```python
from build123d import *

# Parameters (mm, degrees)
SKETCH_1_R          = 8
SKETCH_1_R_2        = 4
EXTRUDE_1_DEPTH     = 3.8
SKETCH_4_W          = 6
SKETCH_4_H          = 6
EXTRUDE_2_DEPTH     = 3.8
SKETCH_5_R          = 2
CUT_EXTRUDE_3_DEPTH = 1
SKETCH_6_R          = 1
CUT_EXTRUDE_4_DEPTH = 15.691494138
CUT_EXTRUDE_5_DEPTH = 15.91442255


with BuildPart() as part:
    # 草图1 → 凸台-拉伸1 (new body)
    with BuildSketch(Plane(origin=(0, 0, 0), x_dir=(1, 0, 0), z_dir=(0, 1, 0))):
        with Locations(Location((0, 0, 0), (0, 0, 90))):
            Circle(SKETCH_1_R)
        with Locations(Location((0, 0, 0), (0, 0, 90))):
            Circle(SKETCH_1_R_2, mode=Mode.SUBTRACT)
    extrude(amount=EXTRUDE_1_DEPTH)

    # 草图4 → 凸台-拉伸2 (add)
    with BuildSketch(Plane(origin=(0, 3.8, 0), x_dir=(1, 0, 0), z_dir=(0, 1, 0))):
        with Locations((-9, 0)):
            Rectangle(SKETCH_4_W, SKETCH_4_H)
        with Locations((9, 0)):
            Rectangle(SKETCH_4_W, SKETCH_4_H)
    extrude(amount=-EXTRUDE_2_DEPTH)

    # 草图5 → 切除-拉伸3 (cut)
    with BuildSketch(Plane.XZ):
        with Locations(Location((-9.5, 0, 0), (0, 0, 270))):
            Circle(SKETCH_5_R)
        with Locations(Location((9.5, 0, 0), (0, 0, 90))):
            Circle(SKETCH_5_R)
    extrude(amount=-CUT_EXTRUDE_3_DEPTH, mode=Mode.SUBTRACT)

    # 草图6 → 切除-拉伸4 (cut, through all)
    with BuildSketch(Plane.XZ.offset(-1)):
        with Locations(Location((-9.5, 0, 0), (0, 0, 270))):
            Circle(SKETCH_6_R)
        with Locations(Location((9.5, 0, 0), (0, 0, 90))):
            Circle(SKETCH_6_R)
    extrude(amount=-CUT_EXTRUDE_4_DEPTH, mode=Mode.SUBTRACT)

    # 草图7 → 切除-拉伸5 (cut, through all)
    with BuildSketch(Plane(origin=(0, 3.8, 0), x_dir=(1, 0, 0), z_dir=(0, 1, 0))):
        with BuildLine():
            Line((-4.05, 6.899094143), (-2.8, 4.734030634))
            Line((-2.8, 4.734030634), (-2.8, 2.856571371))
            ThreePointArc((-2.8, 2.856571371), (0, 4), (2.8, 2.856571371))
            Line((2.8, 2.856571371), (2.8, 4.734030634))
            Line((2.8, 4.734030634), (4.05, 6.899094143))
            ThreePointArc((4.05, 6.899094143), (0, 8), (-4.05, 6.899094143))
        make_face()
    extrude(amount=-CUT_EXTRUDE_5_DEPTH, mode=Mode.SUBTRACT)


solid = part.part
```
Check sheet for the modelled part. Datum: model origin and axes. Units: mm. A direction names the side the tool comes from. Round coordinates to 2 decimals unless told otherwise and drop trailing zeros. Loops run counter-clockwise (first coordinate to the right, second up) from the corner with the lowest first, then second, coordinate; pieces in that order, holes last. Notation, with made-up numbers: (45, 62.25) -> (53, 62.25) arc R15 ccw to (53, 88.25) -> close; hole circle Ø9 at (66.25, -13). An arc over 180 degrees is marked (long way). Write item = value, one per line. Start each with the question number.
1) Sectioned sample at A-A, the plane z = 0. Record the cut outline in (x, y), plus the area to 3 significant figures.
2) Set-up check for faces 1 (the flat face through (-10, 2, -3)), 2 (the flat face through (10, 2, 3)), 3 (the flat face through (-10, 2, 3)): record each of +Z, -Z, +X, -X, +Y, -Y from which the full face is reachable in a straight line by a thin tool's end or side.
3) Sectioned sample at B-B, the plane x = -9.5. Record the cut outline in (y, z).
4) Gauge pin test, flat ends, axial feed: pin 1 Ø1.1 at (x, y) = (10.5, 2) entering from +Z; pin 2 Ø5 at (x, z) = (9.5, 0) entering from +Y; pin 3 Ø2 at (y, z) = (1.5, -4.5) entering from -X; pin 4 Ø1.2 at (x, z) = (9, 0.5) entering from -Y. Record the tip position at first contact, or that the pin passes through.
5) Thickness scan on probe 1 along X at (y, z) = (0.5, 0); probe 2 along X at (y, z) = (2.2, 0); probe 3 along Z at (x, y) = (9.25, 1.55). Record the ranges inside material, lowest first.
6) Sectioned sample at C-C, the plane y = 1.7. Record the cut outline in (x, z).
7) Release check for a two-part mould opening along Z. For faces 4 (the cylindrical face through (0, 2, 4)), 5 (the flat face through (-2.8, 2, -4)), 6 (the flat face through (-10.4, 1, -0.9)), 7 (the flat face through (-3.434, 1.927, -5.832)) record: released by +Z, released by -Z, zero draft, split by the parting line, or undercut.
8) Sectioned sample at D-D, the plane z = -3.75. Record the cut outline in (x, y).
Results are:
q1.outline = (-12, 0) -> (-11.5, 0) -> (-11.5, 1) -> (-10.5, 1) -> (-10.5, 3.8) -> (-12, 3.8) -> close; (-8.5, 1) -> (-7.5, 1) -> (-7.5, 0) -> (-4, 0) -> (-4, 3.8) -> (-8.5, 3.8) -> close; (4, 0) -> (7.5, 0) -> (7.5, 1) -> (8.5, 1) -> (8.5, 3.8) -> (4, 3.8) -> close; (10.5, 1) -> (11.5, 1) -> (11.5, 0) -> (12, 0) -> (12, 3.8) -> (10.5, 3.8) -> close
q1.area = 41.6 mm^2
q2.face_1 = -Z, -X, +Y, -Y
q2.face_2 = +Z, +X, +Y, -Y
q2.face_3 = +Z, -X, +Y, -Y
q3.outline = (0, -3) -> (3.8, -3) -> (3.8, -1) -> (1, -1) -> (1, -2) -> (0, -2) -> close; (0, 2) -> (1, 2) -> (1, 1) -> (3.8, 1) -> (3.8, 3) -> (0, 3) -> close
q4.pin_1 = 3
q4.pin_2 = 3.8
q4.pin_3 = -7.19
q4.pin_4 = 1
q5.probe_1 = -12 to -11.5, -7.5 to -4, 4 to 7.5, 11.5 to 12
q5.probe_2 = -12 to -10.5, -8.5 to -4, 4 to 8.5, 10.5 to 12
q5.probe_3 = -3 to -0.97, 0.97 to 3
q6.outline = (-12, -3) -> (-7.42, -3) arc R8 ccw to (-4.05, -6.9) -> (-2.8, -4.73) -> (-2.8, -2.86) arc R4 cw (long way) to (2.8, -2.86) -> (2.8, -4.73) -> (4.05, -6.9) arc R8 ccw to (7.42, -3) -> (12, -3) -> (12, 3) -> (7.42, 3) arc R8 ccw to (-7.42, 3) -> (-12, 3) -> close; hole circle Ø2 at (-9.5, 0); hole circle Ø2 at (9.5, 0)
q7.face_4 = undercut
q7.face_5 = zero draft
q7.face_6 = undercut
q7.face_7 = released by -Z
q8.outline = (-7.07, 0) -> (-2.8, 0) -> (-2.8, 3.8) -> (-7.07, 3.8) -> close; (2.8, 0) -> (7.07, 0) -> (7.07, 3.8) -> (2.8, 3.8) -> close
